from build123d import *

# Parameters (mm, degrees)
SKETCH026_W             = 122
SKETCH026_H             = 105
PAD006_DEPTH            = 128
SKETCH027_W             = 145.939007
SKETCH027_H             = 190.762029
POCKET019_DEPTH         = 105.001
SKETCH028_W             = 17.5
SKETCH028_H             = 100
SKETCH028_W_2           = 25
SKETCH028_W_3           = 22
POCKET020_DEPTH         = 8.001
SKETCH029_W             = 98.54208
SKETCH029_H             = 3
PAD007_DEPTH            = 7
SKETCH030_R             = 2.25
POCKET021_DEPTH         = 6
SKETCH031_R             = 2.25
POCKET022_DEPTH         = 6
BODY006_PLACEMENT_ANGLE = 180


with BuildPart() as part:
    # Sketch026 → Pad006 (new body)
    with BuildSketch(Plane.XZ):
        with Locations((61, 52.5)):
            Rectangle(SKETCH026_W, SKETCH026_H)
        Polygon((8, 5), (113, 5), (113, 8), (117.5, 8), (117.5, 20.3), (113, 20.3), (113, 40.3), (117.5, 40.3), (117.5, 52.6), (113, 52.6), (113, 72.6), (117.5, 72.6), (117.5, 84.9), (113, 84.9), (113, 100), (8, 100), (8, 84.9), (4, 84.9), (4, 72.6), (8, 72.6), (8, 52.6), (4, 52.6), (4, 40.3), (8, 40.3), (8, 20.3), (4, 20.3), (4, 8), (8, 8), align=None, mode=Mode.SUBTRACT)
    extrude(amount=PAD006_DEPTH)

    # Sketch027 (on Face2 of Pad006) → Pocket019 (cut, through all)
    with BuildSketch(Plane(origin=(0, 0, 105), x_dir=(-1, 0, 0), z_dir=(0, 0, 1))):
        with Locations((-41.0304965, 71.0592985)):
            Rectangle(SKETCH027_W, SKETCH027_H)
    extrude(amount=-POCKET019_DEPTH, mode=Mode.SUBTRACT)

    # Sketch028 (on Face11 of Pocket019) → Pocket020 (cut, through all)
    with BuildSketch(Plane(origin=(114, 0, 0), x_dir=(0, 0, -1), z_dir=(-1, 0, 0))):
        with Locations((-62.75, 65)):
            Rectangle(SKETCH028_W, SKETCH028_H)
        with Locations((-30.25, 65)):
            Rectangle(SKETCH028_W, SKETCH028_H)
        with Locations((-102, 65)):
            Rectangle(SKETCH028_W_2, SKETCH028_H)
        with Locations((4.5, 65)):
            Rectangle(SKETCH028_W_3, SKETCH028_H)
    extrude(amount=-POCKET020_DEPTH, mode=Mode.SUBTRACT)

    # Sketch029 (on Face22 of Pocket020) → Pad007 (join)
    with BuildSketch(Plane(origin=(114, 0, 0), x_dir=(0, 0, -1), z_dir=(-1, 0, 0))):
        with Locations((-51.434969, 126.5)):
            Rectangle(SKETCH029_W, SKETCH029_H)
    extrude(amount=-PAD007_DEPTH)

    # Sketch030 (on Face2 of Pad007) → Pocket021 (cut)
    with BuildSketch(Plane(origin=(0, 0, 0), x_dir=(1, 0, 0), z_dir=(0, 1, 0))):
        with Locations((118, -99)):
            Circle(SKETCH030_R)
        with Locations((118, -67)):
            Circle(SKETCH030_R)
        with Locations((118, -35)):
            Circle(SKETCH030_R)
        with Locations((118, -4)):
            Circle(SKETCH030_R)
    extrude(amount=-POCKET021_DEPTH, mode=Mode.SUBTRACT)

    # Sketch031 (on Face39 of Pocket021) → Pocket022 (cut)
    with BuildSketch(Plane.XZ.offset(128)):
        with Locations((118, 99)):
            Circle(SKETCH031_R)
        with Locations((118, 4)):
            Circle(SKETCH031_R)
    extrude(amount=-POCKET022_DEPTH, mode=Mode.SUBTRACT)


with BuildPart() as part_1:
    # Body006 placement: moved
    add(part.part.moved(Location((126, 0, 0))).rotate(Axis((126, 0, 0), (0, 0, -1)), BODY006_PLACEMENT_ANGLE))


solid = part_1.part
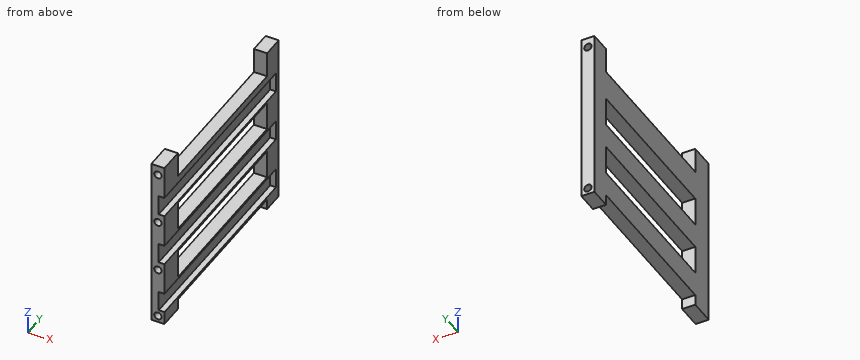
For this review, take the finished solid that the model builds, in its own axes (mm). Round coordinates to 2 decimals unless told otherwise and drop trailing zeros. Loops run counter-clockwise (first coordinate to the right, second up) from the corner with the lowest first, then second, coordinate; pieces in that order, holes last. Notation, with made-up numbers: (72, 7.25) - (129, 7.25) arc R26 cw to (129, 35.25) - close; hole circle Ø2 at (20.5, 66). An arc over 180 degrees is marked (long way). Answer as CSV lines item,"result".
(1) Wall thickness on line 1 (Z direction, x = 8, y = 4); line 2 (Z direction, x = 6.5, y = 50); line 3 (Z direction, x = 9.5, y = 58): over which ranges is each line inside the solid? List them lowest first.
Checked values:
line 1,"z = 0 to 1.75, 6.25 to 32.75, 37.25 to 64.75, 69.25 to 96.75, 101.25 to 105"
line 2,"z = 6.5 to 21.5, 39 to 54, 71.5 to 89.5"
line 3,"z = 6.5 to 8, 20.3 to 21.5, 39 to 40.3, 52.6 to 54, 71.5 to 72.6, 84.9 to 89.5"
(2) Consider section C-C on z = 4. Give the boundary of the cut face in (x, y).
Checked values:
outline,"(4, 0) - (5.75, 0) - (5.75, 6) - (10.25, 6) - (10.25, 0) - (12, 0) - (12, 15) - (4, 15) - close; (4, 115) - (12, 115) - (12, 128) - (10.25, 128) - (10.25, 122) - (5.75, 122) - (5.75, 128) - (4, 128) - close"
(3) Consider section A-A on z = 35. Give the boundary of the cut face in (x, y), then the cut area to 3 significant figures.
Checked values:
outline,"(4, 0) - (5.75, 0) - (5.75, 6) - (10.25, 6) - (10.25, 0) - (12, 0) - (12, 15) - (4, 15) - close; (4, 115) - (12, 115) - (12, 128) - (4, 128) - close"
area,"197 mm2"
(4) Consider section D-D on z = 49. Give the boundary of the cut face in (x, y).
Checked values:
outline,"(4, 0) - (8.5, 0) - (8.5, 125) - (12, 125) - (12, 128) - (4, 128) - close"
(5) Consider section B-B on y = 38. Give the boundary of the cut face in (x, z), then the cut area to 3 significant figures.
Checked values:
outline,"(4, 6.5) - (12, 6.5) - (12, 8) - (8.5, 8) - (8.5, 20.3) - (12, 20.3) - (12, 21.5) - (4, 21.5) - close; (4, 39) - (12, 39) - (12, 40.3) - (8.5, 40.3) - (8.5, 52.6) - (12, 52.6) - (12, 54) - (4, 54) - close; (4, 71.5) - (12, 71.5) - (12, 72.6) - (8.5, 72.6) - (8.5, 84.9) - (12, 84.9) - (12, 89.5) - (4, 89.5) - close"
area,"255 mm2"
(6) Insertion check: P1, Ø1.8, axis at x = 10, y = 64, coming from the +Z side; P2, Ø1.1, axis at x = 10.5, y = 60.5, coming from the -Z side; P3, Ø2, axis at x = 8.5, z = 3, coming from the +Y side. Each pin has a flat end and moves straight along its axis. Give the tip position at first contact, or say it passes through.
Checked values:
P1,"stops at z = 89.5"
P2,"stops at z = 6.5"
P3,"stops at y = 122"
